Check sheet for the modelled part. Datum: model origin and axes. Units: mm. Face numbers are marked on the shaded views. A direction names the side the tool comes from. Round coordinates to 2 decimals unless told otherwise and drop trailing zeros. Write each loop counter-clockwise with the first axis right and the second up, starting at its lowest first coordinate (ties: lowest second). Pieces come first, ordered by that corner, then holes.
Item 1: Depth check by flat-ended pin: pin 1 (3 mm diameter, centred on y = 15.5, z = -15.5, fed in from -X); pin 2 (10 mm diameter, centred on x = -21.5, y = -5.5, fed in from +Z); pin 3 (6.5 mm diameter, centred on x = -9.66, z = 0, fed in from +Y); pin 4 (22 mm diameter, centred on x = -31, z = 1.5, fed in from -Y). Enter the tip coordinate at first touch or a pass-through.
Item 2: Set-up check for the marked faces 1, 2 and 3: record each of +Z, -Z, +X, -X, +Y, -Y from which the full face is reachable in a straight line by a thin tool's end or side.
Item 3: Section check B-B, the plane y = 15.5. State how many separate pieces and enclosed holes the cut face has, plus the area to 3 significant figures.
Item 4: Section check A-A, the plane x = 5.5. Record the cut outline in (y, z).
Item 5: Release check for a two-part mould opening along Y. For the marked faces 4, 5 and 6 record: pulls with the +Y half, pulls with the -Y half, needs draft (parallel to the pull), parting line crosses it, or undercut.
Item 6: Material ranges on line 1 along Y through (x, z) = (30, -13.5); line 2 along Z through (x, y) = (-7, -6), recorded low to high.
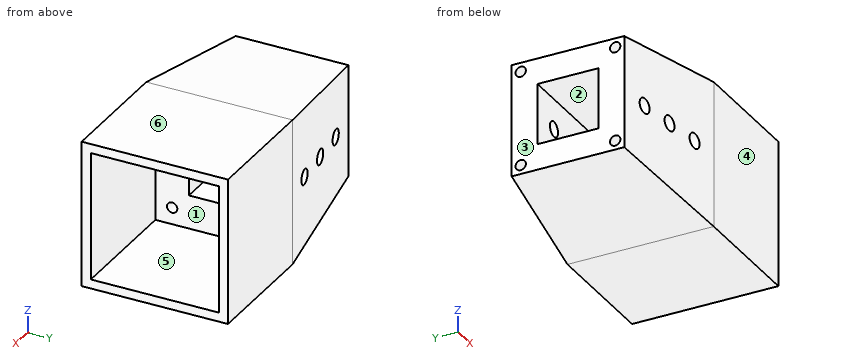
from build123d import *

# Parameters (mm, degrees)
F0_W     = 48
F0_H     = 48
F0_W_2   = 42
F0_H_2   = 42
F0_W_3   = 20
F0_H_3   = 20
F1_DEPTH = 45
F1_TAPER = 7
F2_DEPTH = 60
F3_DEPTH = 40
F4_D     = 3.4
F6_D     = 5
F6_DEPTH = 69
F6_TIP   = 1.5021515476
F7_D     = 5
F7_DEPTH = 69
F7_TIP   = 1.5021515476


with BuildPart() as f1:
    # F0 (on Right) → F1 (new body)
    with BuildSketch(Plane.YZ):
        Rectangle(F0_W, F0_H)
        Rectangle(F0_W_2, F0_H_2, mode=Mode.SUBTRACT)
        Rectangle(F0_W_2, F0_H_2)
        Rectangle(F0_W_3, F0_H_3, mode=Mode.SUBTRACT)
        Rectangle(F0_W_3, F0_H_3)
    extrude(amount=-F1_DEPTH, taper=F1_TAPER)

    # F0 (on Right) → F2 (cut)
    with BuildSketch(Plane.YZ):
        Rectangle(F0_W_3, F0_H_3)
    extrude(amount=-F2_DEPTH, mode=Mode.SUBTRACT)

    # F0 (on Right) → F3 (join)
    with BuildSketch(Plane.YZ):
        Rectangle(F0_W, F0_H)
        Rectangle(F0_W_2, F0_H_2, mode=Mode.SUBTRACT)
    extrude(amount=F3_DEPTH)

    # F4 (through all)
    with Locations(Plane.YZ):
        with Locations((15.5, 15.5), (-15.5, 15.5), (-15.5, -15.5), (15.5, -15.5)):
            Hole(F4_D / 2)

    # F6 (one way)
    with BuildSketch(Plane(origin=(0, -10, 0), x_dir=(-1, 0, 0), z_dir=(0, 1, 0))):
        with Locations((34.7797162831, 0), (22.2414657474, 0), (9.6642384306, 0)):
            Circle(F6_D / 2)
    extrude(amount=-F6_DEPTH, mode=Mode.SUBTRACT)
    with Locations(Plane(origin=(0, -10, 0), x_dir=(-1, 0, 0), z_dir=(0, 1, 0))):
        with Locations((34.7797162831, 0), (22.2414657474, 0), (9.6642384306, 0)):
            with Locations((0, 0, -(F6_DEPTH + F6_TIP / 2))):  # 118° drill point
                Cone(0, F6_D / 2, F6_TIP, mode=Mode.SUBTRACT)

    # F7
    with Locations(Plane(origin=(0, -10, 0), x_dir=(-1, 0, 0), z_dir=(0, -1, 0))):
        with Locations((34.7797162831, 0), (22.2414657474, 0), (9.6642384306, 0)):
            Hole(F7_D / 2, depth=F7_DEPTH)
            with Locations((0, 0, -(F7_DEPTH + F7_TIP / 2))):  # 118° drill point
                Cone(0, F7_D / 2, F7_TIP, mode=Mode.SUBTRACT)


solid = f1.part
Values found:
1. pin 1: passes through
1. pin 2: stops at z = 21.97
1. pin 3: stops at y = 23.21
1. pin 4: stops at y = -21.54
2. face 1: +X
2. face 2: +X, -X
2. face 3: +Z, -Z, -X, +Y, -Y
3. separate pieces: 3
3. enclosed holes: 3
3. area: 1,790 mm2
4. outline: (-24, -24) - (24, -24) - (24, 24) - (-24, 24) - close; hole (-21, -21) - (21, -21) - (21, 21) - (-21, 21) - close
5. face 4: pulls with the -Y half
5. face 5: undercut
5. face 6: needs draft
6. line 1: y = -24 to -21, 21 to 24
6. line 2: z = -23.14 to -10, 10 to 23.14
